Source: CAD feature listing. Evaluate the final solid. Frame: model axes, mm. Face numbers are marked on the shaded views. A direction names the side the tool comes from. Coordinates: 2 decimals unless noted, no trailing zeros. Order: outer loops, then holes, each group sorted by start corner. A loop starts at its lowest first (then second) coordinate and runs counter-clockwise, first axis right, second up. Notation, with made-up numbers: (-4, -14) -> (48, -14) arc R25 cw to (48, 11) -> close; hole circle Ø2 at (57, 30.5). An arc over 180 degrees is marked (long way). Write item = value, one per line. Start each with the question number.
Item 1: Set-up query: the marked faces 3 and 4. Return all of +Z, -Z, +X, -X, +Y, -Y with unobstructed straight access to the full face (end or side cutting, diameter ignored); none if empty.
Item 2: Contact query for flat-ended pins moving along their axis: pin 1 (0.8 mm diameter, centred on y = -3.5, z = 29, fed in from -X); pin 2 (1.2 mm diameter, centred on x = -2.5, y = -1.5, fed in from -Z); pin 3 (1.2 mm diameter, centred on x = -2, y = 0, fed in from +Z); pin 4 (4 mm diameter, centred on y = 2.5, z = 27, fed in from +X). Output: stop coordinate, or through.
Item 3: Mould query, pull axis Y, two halves, no side actions, for the marked faces 1 and 2. Classes: released by +Y, released by -Y, zero draft, split by the parting line, or undercut.
Item 4: Section query C-C (z = 19.5). Output: boundary loops of the cut face in (x, y).
Item 5: Ray query, line 1 along Y through (x, z) = (0, 42); line 2 along Z through (x, y) = (2.5, -2.5). Return the intervals inside material, ascending. Write a range as [from, to].
Item 6: Section query A-A (y = 0). Output: boundary loops of the cut face in (x, z), then the cut area to 3 significant figures.
Item 7: Section query B-B (z = 39.5). Output: boundary loops of the cut face in (x, y), then the cut area to 3 significant figures.
Item 8: Section query D-D (z = 6). Output: boundary loops of the cut face in (x, y), then the cut area to 3 significant figures.
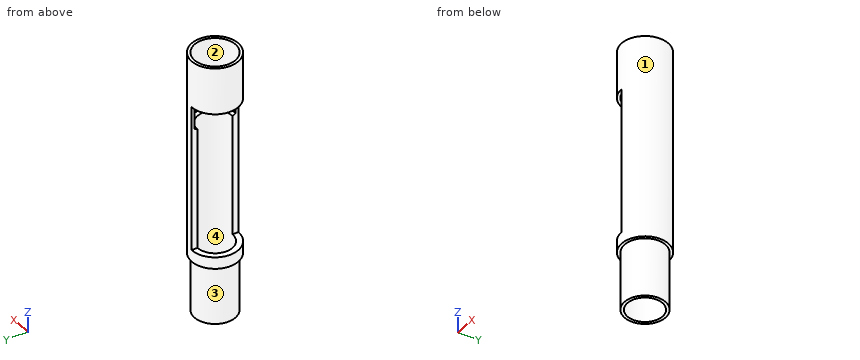
Autodesk Inventor part; units mm, degrees
ref_plane "YZ Plane" through (0, 0, 0) normal (1, 0, 0) x (0, 1, 0)
ref_plane "XZ Plane" through (0, 0, 0) normal (0, 1, 0) x (-1, 0, 0)
ref_plane "XY Plane" through (0, 0, 0) normal (0, 0, 1) x (1, 0, 0)
sketch "Skizze1" plane through (0, 0, 0) normal (0, 0, 1) x (1, 0, 0)
  circle A0 centre (0, 0) radius 4
  circle A1 centre (0, 0) radius 3.5
  dimension "d0" = 8
  dimension "d23" = 7
extrude "Extrusion1" add sketch "Skizze1" along normal blind 45 contours A0 | A1
hole "Bohrung1" at (0, 0, 0) direction (0, 0, 1) diameter 6 end through all
extrude "Extrusion5" cut sketch "Skizze1" along normal blind 10
thread "Gewinde3"
sketch "Skizze5" plane through (0, 0, 45) normal (0, 0, 1) x (1, 0, 0)
  circle A0 centre (0, 0) radius 4
hole "Bohrung2" at (0, 0, 45) direction (0, 0, -1) diameter 7 depth 12 tip angle 118
thread "Gewinde4"
sketch "Skizze6" plane through (0, 0, 0) normal (1, 0, 0) x (0, 1, 0)
  line L0 (5.1203, 12) -> (-6.2581, 12)
  line L1 (-6.2581, 12) -> (-6.2581, 37)
  line L2 (-6.2581, 37) -> (5.1203, 37)
  line L3 (5.1203, 37) -> (5.1203, 12)
  point P0 (0, 0)
  dimension "d37" = 25
extrude "Extrusion6" cut sketch "Skizze6" against normal blind 10
properties part number "PEEKAufsatz1" material "Polyaryletherketon-Kunststoff"
Computed:
q1.face_3 = -Z
q1.face_4 = +Z, -Z
q2.pin_1 = 0
q2.pin_2 = 0
q2.pin_3 = through
q2.pin_4 = 3.97
q3.face_1 = split by the parting line
q3.face_2 = undercut
q4.outline = (0, -4) arc R4 ccw to (0, 4) -> (0, 3) arc R3 cw to (0, -3) -> close
q5.line_1 = [-4, -3.5], [3.5, 4]
q5.line_2 = [10, 45]
q6.outline = (-4, 10) -> (-3.5, 10) -> (-3.5, 0) -> (-3, 0) -> (-3, 12) -> (-4, 12) -> close; (-4, 37) -> (-3.5, 37) -> (-3.5, 45) -> (-4, 45) -> close; (3, 0) -> (3.5, 0) -> (3.5, 10) -> (4, 10) -> (4, 45) -> (3.5, 45) -> (3.5, 33) -> (3, 32.7) -> close
q6.area = 44.9 mm^2
q7.outline = circle Ø8 at (0, 0); hole circle Ø7 at (0, 0)
q7.area = 11.8 mm^2
q8.outline = circle Ø7 at (0, 0); hole circle Ø6 at (0, 0)
q8.area = 10.2 mm^2
